Geometry: see drawing. Coordinates: mm, zero at the bounding-box minimum. A direction names the side the tool comes from. Coordinates: 2 decimals unless noted, no trailing zeros. Write each loop counter-clockwise with the first axis right and the second up, starting at its lowest first coordinate (ties: lowest second). Pieces come first, ordered by that corner, then holes.
1) Section query C-C (y = 9.75). Output: boundary loops of the cut face in (x, z).
2) Section query B-B (x = 6). Output: boundary loops of the cut face in (y, z).
3) Line query: L1, parallel to X at y = 4, z = 3.4; L2, parallel to Z at x = 10.5, y = 7.5. Output: solid intervals per line, ascending.
4) Pin query (flat end, axial travel): pin 1 Ø1.6 at (y, z) = (6, 2) entering from -X; pin 2 Ø2 at (x, z) = (5.5, 3) entering from -Y; pin 3 Ø1 at (y, z) = (4, 2.5) entering from +X. Return the tip coordinate at first contact, or that it passes through.
5) Section query A-A (z = 2.5). Output: boundary loops of the cut face in (x, y).
6) Set-up query: the marked faces 1, 2, 3, 4 and 5. Return all of +Z, -Z, +X, -X, +Y, -Y with unobstructed straight access to the full face (end or side cutting, diameter ignored); none if empty.
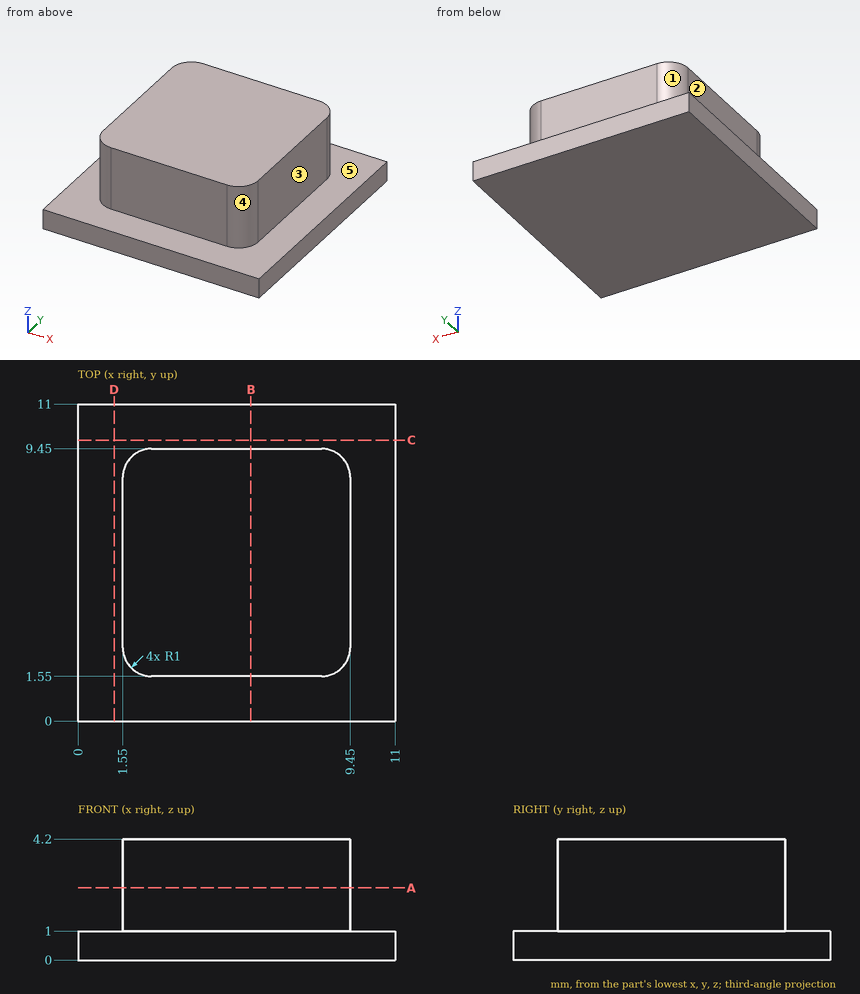
Answer:
1. outline: (0, 0) - (11, 0) - (11, 1) - (0, 1) - close
2. outline: (0, 0) - (11, 0) - (11, 1) - (9.45, 1) - (9.45, 4.2) - (1.55, 4.2) - (1.55, 1) - (0, 1) - close
3. L1: x = 1.55 to 9.45
3. L2: z = 0 to 1
4. pin 1: stops at x = 1.55
4. pin 2: stops at y = 1.55
4. pin 3: stops at x = 9.45
5. outline: (1.55, 2.55) arc R1 ccw to (2.55, 1.55) - (8.45, 1.55) arc R1 ccw to (9.45, 2.55) - (9.45, 8.45) arc R1 ccw to (8.45, 9.45) - (2.55, 9.45) arc R1 ccw to (1.55, 8.45) - close
6. face 1: +Z, -X, +Y
6. face 2: +Z, -X, +Y, -Y
6. face 3: +Z, +X, +Y, -Y
6. face 4: +Z, +X, -Y
6. face 5: +Z
